Geometry check sheet. Reference: the model listing, model coordinates, mm. A direction names the side the tool comes from. Give positions to 0.01 mm unless a question says otherwise; leave off trailing zeros. Loops run counter-clockwise (first coordinate to the right, second up) from the corner with the lowest first, then second, coordinate; pieces in that order, holes last. Notation, with made-up numbers: (69.5, 51) - (104.5, 51) arc R14 ccw to (104.5, 70) - close; hole circle Ø6 at (-29, 48.25). An arc over 180 degrees is marked (long way). Use a Markdown table: item, result. Add a question column.
1. Depth check by flat-ended pin: P1, Ø11.5, axis at x = 0, z = 0, coming from the -Y side; P2, Ø5.5, axis at x = 0.5, z = -1, coming from the +Y side; P3, Ø4, axis at x = 7.5, z = -5.5, coming from the -Y side; P4, Ø1, axis at y = 7.5, z = 9.5, coming from the -X side. Enter the tip coordinate at first touch or a pass-through.
2. Set-up check for faces 1 (the cylindrical face through (-13.948, 5.91, -3.097)), 2 (the cylindrical face through (-3.5, 4.43, -0.46)), 3 (the cylindrical face through (3.86, -3.35, -5.04)), 4 (the flat face through (8, 6.985, 0)): record each of +Z, -Z, +X, -X, +Y, -Y from which the full face is reachable in a straight line by a thin tool's end or side.
3. Cross-section at C-C on y = 7.5. Enter the section's corners in (x, z) (1 decimal).
4. Cross-section at D-D on y = -2.5. Enter the section's corners in (x, z).
5. Cross-section at B-B on z = 0. Count the separate pieces of the cut face and the enclosed holes in it, and give its area (3 significant figures).
6. Material ranges on L1, parallel to X at y = 3.75, z = 0; L2, parallel to X at y = 0.25, z = 4.5; L3, parallel to X at y = -1.65, z = 0, recorded low to high.
7. Draft check along Z on faces 5 (the conical face through (-0.148, 15.131, 14.014)), 6 (the cylindrical face through (-0.767, -2.817, 2.435)), 7 (the flat face through (0, 15.24, 12)). Enter one of: pulls with the +Z half, pulls with the -Z half, needs draft (parallel to the pull), parting line crosses it, or undercut.
from build123d import *

# Parameters (mm, degrees)
SKETCH1_R               = 14.2875
EXTRUDE1_DEPTH          = 15.24
CUT_EXTRUDE1_DEPTH      = 15.2875
CUT_EXTRUDE1_DEPTH_BACK = 15.2875
SKETCH6_R               = 6.35
EXTRUDE2_DEPTH          = 6.35
CHAMFER1_SIZE           = 0.6223
CHAMFER2_SIZE           = 0.381
SKETCH8_R               = 0.635
SKETCH9_R               = 1.1811
CUT_EXTRUDE2_DEPTH      = 14.335


with BuildPart() as part:
    # Sketch1 → Extrude1 (new body)
    with BuildSketch(Plane(origin=(0, 0, 0), x_dir=(1, 0, 0), z_dir=(0, 1, 0))):
        with Locations(Location((0, 0, 0), (0, 0, 270))):  # turned: the seam where the file's is
            Circle(SKETCH1_R)
    extrude(amount=EXTRUDE1_DEPTH)

    # Sketch3 → Cut-Extrude1 (cut, two sides)
    with BuildSketch(Plane(origin=(0, 0, 0), x_dir=(0, 0, -1), z_dir=(1, 0, 0))) as cut_extrude1_sk:
        Polygon((-10.803384182, 15.24), (10.803384182, 15.24), (2.548384182, 6.985), (-2.548384182, 6.985), align=None)
    extrude(amount=CUT_EXTRUDE1_DEPTH, mode=Mode.SUBTRACT)
    extrude(cut_extrude1_sk.sketch, amount=-CUT_EXTRUDE1_DEPTH_BACK, mode=Mode.SUBTRACT)

    # Sketch6 → Extrude2 (add)
    with BuildSketch(Plane.XZ):
        with Locations(Location((0, 0, 0), (0, 0, 90))):  # turned: the seam where the file's is
            Circle(SKETCH6_R)
    extrude(amount=EXTRUDE2_DEPTH)

    # Sketch7 → Cut-Revolve1 (revolve, cut)
    with BuildSketch(Plane.XY, mode=Mode.PRIVATE) as cut_revolve1_sk:
        Polygon((0, -6.35), (2.5527, -6.35), (2.5527, 0.635), (3.5306, 0.635), (3.5306, 6.985), (3.5306, 15.24), (0, 15.24), (0, 6.985), align=None)
    revolve(cut_revolve1_sk.sketch.rotate(Axis((0, 13.979393491, 0), (0, -1, 0)), 90), axis=Axis((0, 13.979393491, 0), (0, -1, 0)), mode=Mode.SUBTRACT)  # turned: the seam where the file's is

    # Chamfer1
    chamfer1_edges = [part.edges().sort_by_distance(p)[0] for p in [
        (0, -6.35, -2.5527),
        (0, 0.635, -2.5527),
    ]]
    chamfer(chamfer1_edges, length=CHAMFER1_SIZE)

    # Chamfer2
    chamfer2_edges = [part.edges().sort_by_distance(p)[0] for p in [
        (0, 15.24, -14.2875),
        (-4.988953034, 15.24, 13.388166561),
        (0, 0, -14.2875),
        (0, -6.35, -6.35),
    ]]
    chamfer(chamfer2_edges, length=CHAMFER2_SIZE)

    # Sketch8 → Cut-Revolve2 (revolve, cut)
    with BuildSketch(Plane.XY, mode=Mode.PRIVATE) as cut_revolve2_sk:
        with Locations((6.6675, -0.254)):
            Circle(SKETCH8_R)
    revolve(cut_revolve2_sk.sketch.rotate(Axis((0, 0, 0), (0, -1, 0)), 90), axis=Axis((0, 0, 0), (0, -1, 0)), mode=Mode.SUBTRACT)  # turned: the seam where the file's is

    # Sketch9 → Cut-Extrude2 (cut, through all)
    with BuildSketch(Plane(origin=(0, 6.985, 0), x_dir=(-1, 0, 0), z_dir=(0, 1, 0))):
        with Locations(Location((-10.16, 0, 0), (0, 0, 90))):  # turned: the seam where the file's is
            Circle(SKETCH9_R)
    extrude(amount=-CUT_EXTRUDE2_DEPTH, mode=Mode.SUBTRACT)


solid = part.part
Values found:
| question | item | result |
|---|---|---|
| 1 | P1 | stops at y = -6.35 |
| 1 | P2 | stops at y = 8.19 |
| 1 | P3 | stops at y = 0 |
| 1 | P4 | stops at x = -11.1 |
| 2 | face 1 | +Y, -Y |
| 2 | face 2 | +Y |
| 2 | face 3 | -Y |
| 2 | face 4 | +X, -X, +Y |
| 3 | outline | (-14, -3.1) arc R14.3 ccw to (14, -3.1) - (1.8, -3.1) arc R3.5 cw to (-1.8, -3.1) - close; (-14, 3.1) - (-1.8, 3.1) arc R3.5 cw to (1.8, 3.1) - (14, 3.1) arc R14.3 ccw to start |
| 4 | outline | circle Ø12.7 at (0, 0); hole circle Ø5.11 at (0, 0) |
| 5 | separate pieces | 3 |
| 5 | enclosed holes | 0 |
| 5 | area | 181 mm2 |
| 6 | L1 | x = -14.29 to -3.53, 3.53 to 8.98, 11.34 to 14.29 |
| 6 | L2 | x = -13.42 to -5.43, -4.38 to 4.38, 5.43 to 13.42 |
| 6 | L3 | x = -6.35 to -2.55, 2.55 to 6.35 |
| 7 | face 5 | pulls with the +Z half |
| 7 | face 6 | undercut |
| 7 | face 7 | needs draft |
